Build history of the part. All positions in model axes, mm. Face numbers are marked on the shaded views. Round coordinates to 2 decimals unless told otherwise and drop trailing zeros. Loops run counter-clockwise (first coordinate to the right, second up) from the corner with the lowest first, then second, coordinate; pieces in that order, holes last. Notation, with made-up numbers: (-37.5, -30.75) - (16.5, -30.75) arc R20 cw to (16.5, -6.75) - close; hole circle Ø1 at (63, -19.75). An arc over 180 degrees is marked (long way). Use a Markdown table: item, result.
Autodesk Inventor part; units mm, degrees
ref_plane "YZ Plane" through (0, 0, 0) normal (1, 0, 0) x (0, 1, 0)
ref_plane "XZ Plane" through (0, 0, 0) normal (0, 1, 0) x (-1, 0, 0)
ref_plane "XY Plane" through (0, 0, 0) normal (0, 0, 1) x (1, 0, 0)
sketch "Sketch1" plane through (0, 0, 0) normal (0, 1, 0) x (-1, 0, 0)
  circle A0 centre (0, 0) radius 10.5
  line L0 (0, 0) -> (0, -23.5)
  circle A1 centre (0, -23.5) radius 5.25
  line L1 (0, -23.5) -> (0, -35.25)
  line L2 (-14, -35.25) -> (-14, -58.75)
  line L3 (-14, -58.75) -> (-19, -58.75)
  line L4 (-19, -58.75) -> (-19, -35.25)
  line L5 (-35.25, 21.625) -> (35.25, 21.625)
  line L6 (-35.25, 21.625) -> (35.25, 21.625) construction
  line L7 (35.25, 21.625) -> (25.25, 21.625)
  line L8 (-35.25, 21.625) -> (35.25, 21.625)
  line L9 (35.25, 21.625) -> (35.25, -69.875)
  line L10 (35.25, -69.875) -> (-35.25, -69.875)
  line L11 (-35.25, -69.875) -> (-35.25, 21.625)
  line L12 (-35.25, 21.625) -> (-35.25, 11.625)
  line L13 (-35.25, 11.625) -> (-25.25, 11.625)
  circle A2 centre (-25.25, 11.625) radius 3.5
  line L14 (35.25, 21.625) -> (25.25, 21.625)
  line L15 (25.25, 21.625) -> (25.25, 11.625)
  circle A3 centre (25.25, 11.625) radius 3.5
  line L16 (35.25, -69.875) -> (25.25, -69.875)
  line L17 (25.25, -69.875) -> (25.25, -59.875)
  circle A4 centre (25.25, -59.875) radius 3.5
  line L18 (-35.25, -69.875) -> (-25.25, -69.875)
  line L19 (-25.25, -69.875) -> (-25.25, -59.875)
  circle A5 centre (-25.25, -59.875) radius 3.5
  line L20 (-25.25, 11.625) -> (-25.25, -18.375)
  line L21 (25.25, -59.875) -> (25.25, -29.875)
  circle A6 centre (-25.25, -18.375) radius 2.5
  circle A7 centre (25.25, -29.875) radius 2.5
  line L22 (-19, -35.25) -> (-14, -35.25)
  dimension "d0" = 21
  dimension "d1" = 23.5
  dimension "d2" = 10.5
  dimension "d3" = 11.75
  dimension "d5" = 23.5
  dimension "d6" = 5
  dimension "d7" = 23.5
  dimension "d9" = 70.5
  dimension "d40" = 21.625
  dimension "d41" = 70.5
  dimension "d42" = 91.5
  dimension "d43" = 10
  dimension "d44" = 10
  dimension "d45" = 7
  dimension "d46" = 10
  dimension "d47" = 10
  dimension "d48" = 90
  dimension "d50" = 7
  dimension "d51" = 10
  dimension "d52" = 10
  dimension "d53" = 7
  dimension "d54" = 10
  dimension "d55" = 10
  dimension "d56" = 7
  dimension "d60" = 30
  dimension "d61" = 30
  dimension "d62" = 5
  dimension "d63" = 5
  dimension "d64" = 14
extrude "Extrusion1" add sketch "Sketch1" along normal blind 20
hole "Hole1" at (0, 0, 0) direction (0, 1, 0) diameter 3 end through all counterbore diameter 25 counterbore depth 3
hole "Hole2" at (0, 0, -23.5) direction (0, 1, 0) diameter 3 end through all counterbore diameter 14.5 counterbore depth 3
sketch "Sketch2" plane through (0, 0, 0) normal (0, -1, 0) x (1, 0, 0)
  line L0 (12, -33.25) -> (21, -33.25)
  line L1 (21, -33.25) -> (21, -61)
  line L2 (21, -61) -> (12, -61)
  line L3 (12, -61) -> (12, -33.25)
  point P0 (0, 0)
  dimension "d85" = 33.25
  dimension "d86" = 12
  dimension "d87" = 9
  dimension "d88" = 27.75
extrude "Extrusion2" cut sketch "Sketch2" against normal blind 3
properties part number "Guia"
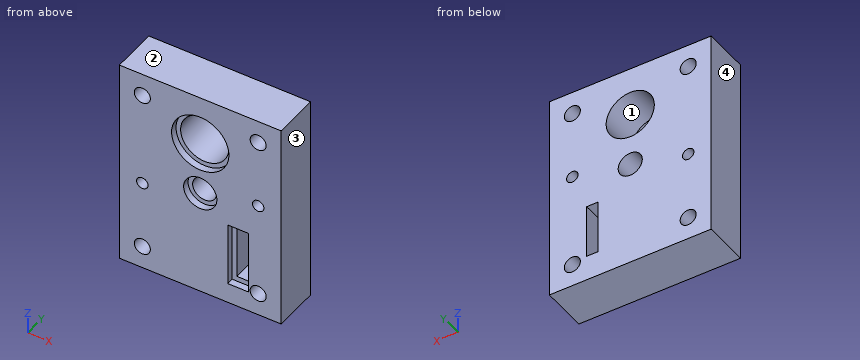
Q1. Cut at D-D, the plane x = 0. List the corners of the cut face in (y, z) (3 decimals).
Results found:
| item | result |
|---|---|
| outline | (0, -69.875) - (20, -69.875) - (20, -28.75) - (3, -28.75) - (3, -30.75) - (0, -30.75) - close; (0, -16.25) - (3, -16.25) - (3, -18.25) - (20, -18.25) - (20, -10.5) - (3, -10.5) - (3, -12.5) - (0, -12.5) - close; (0, 12.5) - (3, 12.5) - (3, 10.5) - (20, 10.5) - (20, 21.625) - (0, 21.625) - close |
Q2. Cut at A-A, the plane x = 17. List the corners of the cut face in (y, z) (3 decimals), plus the area to 3 significant figures.
Results found:
| item | result |
|---|---|
| outline | (0, -69.875) - (20, -69.875) - (20, -58.75) - (3, -58.75) - (3, -61) - (0, -61) - close; (0, -33.25) - (3, -33.25) - (3, -35.25) - (20, -35.25) - (20, 21.625) - (0, 21.625) - close |
| area | 1,350 mm2 |
Q3. Drop flat-ended pins along their axis: pin 1 (5.5 mm diameter, centred on x = 25.25, z = -59.875, fed in from -Y) (3 decimals); pin 2 (4 mm diameter, centred on x = 3, z = -9, fed in from -Y); pin 3 (8 mm diameter, centred on x = 25.25, z = 11.625, fed in from -Y). Give the stop position or say it passes through.
Results found:
| item | result |
|---|---|
| pin 1 | passes through |
| pin 2 | stops at y = 3 |
| pin 3 | stops at y = 0 |
Q4. Cut at B-B, the plane z = 0. List the corners of the cut face in (x, y), plus the area to 3 significant figures.
Results found:
| item | result |
|---|---|
| outline | (-35.25, 0) - (-12.5, 0) - (-12.5, 3) - (-10.5, 3) - (-10.5, 20) - (-35.25, 20) - close; (10.5, 3) - (12.5, 3) - (12.5, 0) - (35.25, 0) - (35.25, 20) - (10.5, 20) - close |
| area | 978 mm2 |
Q5. Probe line 1 (Z direction, x = 25.25, y = 8.25) (3 decimals); line 2 (X direction, y = 1.2, z = -23.5); line 3 (Z direction, x = -23, y = 2) (3 decimals). List the from-to ranges inside material, lowest first.
Results found:
| item | result |
|---|---|
| line 1 | z = -69.875 to -63.375, -56.375 to -20.875, -15.875 to 8.125, 15.125 to 21.625 |
| line 2 | x = -35.25 to -7.25, 7.25 to 35.25 |
| line 3 | z = -69.875 to -62.556, -57.194 to -30.965, -28.785 to 8.944, 14.306 to 21.625 |
Q6. Cut at C-C, the plane x = 25.25. List the corners of the cut face in (y, z) (3 decimals), plus the area to 3 significant figures.
Results found:
| item | result |
|---|---|
| outline | (0, -69.875) - (20, -69.875) - (20, -63.375) - (0, -63.375) - close; (0, -56.375) - (20, -56.375) - (20, -20.875) - (0, -20.875) - close; (0, -15.875) - (20, -15.875) - (20, 8.125) - (0, 8.125) - close; (0, 15.125) - (20, 15.125) - (20, 21.625) - (0, 21.625) - close |
| area | 1,450 mm2 |
Q7. Pull direction X, two halves, no side cores. Call the marked faces 1, 2, 3 and 4: pulls with the +X half, pulls with the -X half, needs draft (parallel to the pull), parting line crosses it, or undercut.
Results found:
| item | result |
|---|---|
| face 1 | undercut |
| face 2 | needs draft |
| face 3 | pulls with the +X half |
| face 4 | pulls with the -X half |
